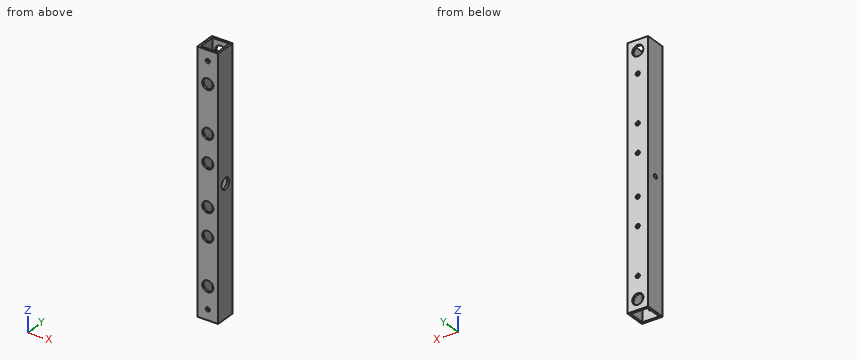
from build123d import *

# Parameters (mm, degrees)
SKETCH_1_W           = 15
SKETCH_1_H           = 15
SKETCH_1_W_2         = 12
SKETCH_1_H_2         = 12
EXTRUDE_2_DEPTH      = 185
SKETCH_2_R           = 4
CUT_EXTRUDE_1_DEPTH  = 10
SKETCH_3_R           = 1.5
CUT_EXTRUDE_2_DEPTH  = 10
SKETCH_4_R           = 4
CUT_EXTRUDE_3_DEPTH  = 10
SKETCH_5_R           = 1.5
CUT_EXTRUDE_4_DEPTH  = 10
SKETCH_6_R           = 1.5
CUT_EXTRUDE_5_DEPTH  = 10
SKETCH_7_R           = 4
CUT_EXTRUDE_6_DEPTH  = 10
SKETCH_8_R           = 1.5
CUT_EXTRUDE_7_DEPTH  = 10
SKETCH_9_R           = 1.5
CUT_EXTRUDE_8_DEPTH  = 10
SKETCH_10_R          = 4
CUT_EXTRUDE_9_DEPTH  = 10
SKETCH_11_R          = 4
CUT_EXTRUDE_10_DEPTH = 10
SKETCH_12_R          = 1.5
CUT_EXTRUDE_11_DEPTH = 10
SKETCH_14_R          = 1.5
CUT_EXTRUDE_12_DEPTH = 10
SKETCH_15_R          = 4
CUT_EXTRUDE_13_DEPTH = 10
SKETCH_16_R          = 4
CUT_EXTRUDE_14_DEPTH = 10
SKETCH_18_R          = 1.5
CUT_EXTRUDE_15_DEPTH = 10
SKETCH_19_R          = 1.5
CUT_EXTRUDE_16_DEPTH = 10
SKETCH_20_R          = 4
CUT_EXTRUDE_17_DEPTH = 10
SKETCH_21_R          = 4
CUT_EXTRUDE_18_DEPTH = 10


with BuildPart() as part:
    # ｽｹｯﾁ1 → ﾎﾞｽ - 押し出し2 (new body)
    with BuildSketch(Plane.XY):
        with Locations((0.489915859, 0.232626086)):
            Rectangle(SKETCH_1_W, SKETCH_1_H)
        with Locations((0.489915859, 0.232626086)):
            Rectangle(SKETCH_1_W_2, SKETCH_1_H_2, mode=Mode.SUBTRACT)
    extrude(amount=EXTRUDE_2_DEPTH)

    # ｽｹｯﾁ2 → ｶｯﾄ - 押し出し1 (cut)
    with BuildSketch(Plane(origin=(0, 7.732626086, 0), x_dir=(1, 0, 0), z_dir=(0, 1, 0))):
        with Locations((0.489915859, -177.5)):
            Circle(SKETCH_2_R)
    extrude(amount=-CUT_EXTRUDE_1_DEPTH, mode=Mode.SUBTRACT)

    # ｽｹｯﾁ3 → ｶｯﾄ - 押し出し2 (cut)
    with BuildSketch(Plane.XZ.offset(7.267373914)):
        with Locations((0.489915859, 177.5)):
            Circle(SKETCH_3_R)
    extrude(amount=-CUT_EXTRUDE_2_DEPTH, mode=Mode.SUBTRACT)

    # ｽｹｯﾁ4 → ｶｯﾄ - 押し出し3 (cut)
    with BuildSketch(Plane(origin=(0, 7.732626086, 0), x_dir=(1, 0, 0), z_dir=(0, 1, 0))):
        with Locations((0.489915859, -7.5)):
            Circle(SKETCH_4_R)
    extrude(amount=-CUT_EXTRUDE_3_DEPTH, mode=Mode.SUBTRACT)

    # ｽｹｯﾁ5 → ｶｯﾄ - 押し出し4 (cut)
    with BuildSketch(Plane.XZ.offset(7.267373914)):
        with Locations((0.489915859, 7.5)):
            Circle(SKETCH_5_R)
    extrude(amount=-CUT_EXTRUDE_4_DEPTH, mode=Mode.SUBTRACT)

    # ｽｹｯﾁ6 → ｶｯﾄ - 押し出し5 (cut)
    with BuildSketch(Plane.ZY.offset(7.010084141)):
        with Locations((92.5, 0.232626086)):
            Circle(SKETCH_6_R)
    extrude(amount=-CUT_EXTRUDE_5_DEPTH, mode=Mode.SUBTRACT)

    # ｽｹｯﾁ7 → ｶｯﾄ - 押し出し6 (cut)
    with BuildSketch(Plane(origin=(7.989915859, 0, 0), x_dir=(0, 0, -1), z_dir=(1, 0, 0))):
        with Locations((-92.5, 0.232626086)):
            Circle(SKETCH_7_R)
    extrude(amount=-CUT_EXTRUDE_6_DEPTH, mode=Mode.SUBTRACT)

    # ｽｹｯﾁ8 → ｶｯﾄ - 押し出し7 (cut)
    with BuildSketch(Plane(origin=(0, 7.732626086, 0), x_dir=(1, 0, 0), z_dir=(0, 1, 0))):
        with Locations((0.489915859, -77.5)):
            Circle(SKETCH_8_R)
    extrude(amount=-CUT_EXTRUDE_7_DEPTH, mode=Mode.SUBTRACT)

    # ｽｹｯﾁ9 → ｶｯﾄ - 押し出し8 (cut)
    with BuildSketch(Plane(origin=(0, 7.732626086, 0), x_dir=(1, 0, 0), z_dir=(0, 1, 0))):
        with Locations((0.489915859, -107.5)):
            Circle(SKETCH_9_R)
    extrude(amount=-CUT_EXTRUDE_8_DEPTH, mode=Mode.SUBTRACT)

    # ｽｹｯﾁ10 → ｶｯﾄ - 押し出し9 (cut)
    with BuildSketch(Plane.XZ.offset(7.267373914)):
        with Locations((0.489915859, 77.5)):
            Circle(SKETCH_10_R)
    extrude(amount=-CUT_EXTRUDE_9_DEPTH, mode=Mode.SUBTRACT)

    # ｽｹｯﾁ11 → ｶｯﾄ - 押し出し10 (cut)
    with BuildSketch(Plane.XZ.offset(7.267373914)):
        with Locations((0.489915859, 107.5)):
            Circle(SKETCH_11_R)
    extrude(amount=-CUT_EXTRUDE_10_DEPTH, mode=Mode.SUBTRACT)

    # ｽｹｯﾁ12 → ｶｯﾄ - 押し出し11 (cut)
    with BuildSketch(Plane(origin=(0, 7.732626086, 0), x_dir=(1, 0, 0), z_dir=(0, 1, 0))):
        with Locations((0.489915859, -23.3)):
            Circle(SKETCH_12_R)
    extrude(amount=-CUT_EXTRUDE_11_DEPTH, mode=Mode.SUBTRACT)

    # ｽｹｯﾁ14 → ｶｯﾄ - 押し出し12 (cut)
    with BuildSketch(Plane(origin=(0, 7.732626086, 0), x_dir=(1, 0, 0), z_dir=(0, 1, 0))):
        with Locations((0.489915859, -57.3)):
            Circle(SKETCH_14_R)
    extrude(amount=-CUT_EXTRUDE_12_DEPTH, mode=Mode.SUBTRACT)

    # ｽｹｯﾁ15 → ｶｯﾄ - 押し出し13 (cut)
    with BuildSketch(Plane.XZ.offset(7.267373914)):
        with Locations((0.489915859, 23.3)):
            Circle(SKETCH_15_R)
    extrude(amount=-CUT_EXTRUDE_13_DEPTH, mode=Mode.SUBTRACT)

    # ｽｹｯﾁ16 → ｶｯﾄ - 押し出し14 (cut)
    with BuildSketch(Plane.XZ.offset(7.267373914)):
        with Locations((0.489915859, 57.3)):
            Circle(SKETCH_16_R)
    extrude(amount=-CUT_EXTRUDE_14_DEPTH, mode=Mode.SUBTRACT)

    # ｽｹｯﾁ18 → ｶｯﾄ - 押し出し15 (cut)
    with BuildSketch(Plane(origin=(0, 7.732626086, 0), x_dir=(1, 0, 0), z_dir=(0, 1, 0))):
        with Locations((0.489915859, -161.7)):
            Circle(SKETCH_18_R)
    extrude(amount=-CUT_EXTRUDE_15_DEPTH, mode=Mode.SUBTRACT)

    # ｽｹｯﾁ19 → ｶｯﾄ - 押し出し16 (cut)
    with BuildSketch(Plane(origin=(0, 7.732626086, 0), x_dir=(1, 0, 0), z_dir=(0, 1, 0))):
        with Locations((0.489915859, -127.7)):
            Circle(SKETCH_19_R)
    extrude(amount=-CUT_EXTRUDE_16_DEPTH, mode=Mode.SUBTRACT)

    # ｽｹｯﾁ20 → ｶｯﾄ - 押し出し17 (cut)
    with BuildSketch(Plane.XZ.offset(7.267373914)):
        with Locations((0.489915859, 161.7)):
            Circle(SKETCH_20_R)
    extrude(amount=-CUT_EXTRUDE_17_DEPTH, mode=Mode.SUBTRACT)

    # ｽｹｯﾁ21 → ｶｯﾄ - 押し出し18 (cut)
    with BuildSketch(Plane(origin=(0, -7.267373914, 0), x_dir=(-1, 0, 0), z_dir=(0, -1, 0))):
        with Locations((-0.489915859, -127.7)):
            Circle(SKETCH_21_R)
    extrude(amount=-CUT_EXTRUDE_18_DEPTH, mode=Mode.SUBTRACT)


solid = part.part
Input: part model. Units: mm. Frame: model coordinates. Give positions to 0.01 mm unless a question says otherwise; leave off trailing zeros. Order: outer loops, then holes, each group sorted by start corner. A loop starts at its lowest first (then second) coordinate and runs counter-clockwise, first axis right, second up.
Q1. Contact query for flat-ended pins moving along their axis: pin 1 Ø2.5 at (x, z) = (0.49, 161.7) entering from -Y; pin 2 Ø4 at (y, z) = (0.23, 92.5) entering from +X; pin 3 Ø4 at (x, z) = (0.49, 107.5) entering from -Y. Output: stop coordinate, or through.
Checked values:
pin 1: passes through
pin 2: stops at x = -5.51
pin 3: stops at y = 6.23
Q2. Section B-B on z = 46. Output: boundary loops of the cut face in (x, y).
Checked values:
outline: (-7.01, -7.27) - (7.99, -7.27) - (7.99, 7.73) - (-7.01, 7.73) - close; hole (-5.51, -5.77) - (6.49, -5.77) - (6.49, 6.23) - (-5.51, 6.23) - close
Q3. Section A-A on z = 23.3. Output: boundary loops of the cut face in (x, y), and give its area (3 significant figures).
Checked values:
outline: (-7.01, -7.27) - (-3.51, -7.27) - (-3.51, -5.77) - (-5.51, -5.77) - (-5.51, 6.23) - (-1.01, 6.23) - (-1.01, 7.73) - (-7.01, 7.73) - close; (1.99, 6.23) - (6.49, 6.23) - (6.49, -5.77) - (4.49, -5.77) - (4.49, -7.27) - (7.99, -7.27) - (7.99, 7.73) - (1.99, 7.73) - close
area: 64.5 mm2
Q4. Ray query, probe 1 along X at (y, z) = (3.5, 124); probe 2 along Y at (x, z) = (-3, 119.5); probe 3 along X at (y, z) = (6.8, 57.3). Return the intervals inside material, ascending.
Checked values:
probe 1: x = -7.01 to -5.51, 6.49 to 7.99
probe 2: y = -7.27 to -5.77, 6.23 to 7.73
probe 3: x = -7.01 to -1.01, 1.99 to 7.99
